Could you check a few things on this model? Use its own coordinates, in mm. A direction names the side the tool comes from. Give positions to 0.01 mm unless a question says otherwise; leave off trailing zeros. Order: outer loops, then holes, each group sorted by start corner. A loop starts at its lowest first (then second) coordinate and runs counter-clockwise, first axis right, second up. Notation, with made-up numbers: (23.25, -3.75) - (75.25, -3.75) arc R18 ccw to (75.25, 11.25) - close; hole circle Ø10 at (69, -0.75). An arc over 180 degrees is marked (long way). One line per question, with ' | ' between items. Start each with the question number.
1. If we mould it in two halves opening along X, with no side actions, what happens to faces 1 (the flat face through (5, -40, 5)), 2 (the flat face through (0, -12.5, 5)), 3 (the flat face through (0, -19, 10))? For each: released by +X, released by -X, zero draft, split by the parting line, or undercut.
2. Imagine slicing it at D-D (y = -54). Please give me the cut outline in (x, z), and give its area (3 significant figures).
3. Imagine slicing it at B-B (x = 0). Please give me the cut outline in (y, z), and give its area (3 significant figures).
4. Which directions (+Z, -Z, +X, -X, +Y, -Y) give clear straight access to the entire face, cutting with the end or side of a thin tool? Please do faces 4 (the flat face through (-5, -39, 5)), 5 (the flat face through (0, -59.365, 5)), 6 (the flat face through (2.5, -11, 5)).
5. I need wall thicknesses on probe 1 along Y at (x, z) = (0, 6.25); probe 2 along X at (y, z) = (-37.5, 9); probe 3 along X at (y, z) = (0, 6.25). Which ranges of each line are inside material? Lowest first, please. Write a range as from..to.
6. Imagine slicing it at C-C (z = 3.25). Please give me the cut outline in (x, y).
7. Imagine slicing it at A-A (y = 0). Please give me the cut outline in (x, z), and give its area (3 significant figures).
8. For P1, Ø6, axis at x = -14, z = 7.5, coming from the +Y side; P2, Ø0.8, axis at y = -11, z = 4, coming from the +X side; P3, Ø12, axis at x = 0, y = 0, coming from the +Z side; P4, Ø3, axis at y = -11, z = 4, coming from the -X side, each with a flat end and sliding along its axis, tell me the tip position at first contact or that it passes through.
```python
from build123d import *

# Parameters (mm, degrees)
BOSS_EXTRUDE1_DEPTH = 10


with BuildPart() as part:
    # Sketch1 → Boss-Extrude1 (new body)
    with BuildSketch(Plane.XY):
        with BuildLine():
            Line((-5, -59.364916731), (5, -59.364916731))
            Line((5, -59.364916731), (5, -19.364916731))
            ThreePointArc((5, -19.364916731), (0, 20), (-5, -19.364916731))
            Line((-5, -19.364916731), (-5, -59.364916731))
        make_face()
        with BuildLine():
            Line((-2.5, -12.5), (2.5, -12.5))
            Line((2.5, -12.5), (2.5, -9.682458366))
            ThreePointArc((2.5, -9.682458366), (0, 10), (-2.5, -9.682458366))
            Line((-2.5, -9.682458366), (-2.5, -12.5))
        make_face(mode=Mode.SUBTRACT)
    extrude(amount=BOSS_EXTRUDE1_DEPTH)


solid = part.part
```
Results found:
1) face 1: released by +X | face 2: undercut | face 3: zero draft
2) outline: (-5, 0) - (5, 0) - (5, 10) - (-5, 10) - close | area: 100 mm2
3) outline: (-59.36, 0) - (-12.5, 0) - (-12.5, 10) - (-59.36, 10) - close; (10, 0) - (20, 0) - (20, 10) - (10, 10) - close | area: 569 mm2
4) face 4: +Z, -Z, -X, -Y | face 5: +Z, -Z, +X, -X, -Y | face 6: +Z, -Z
5) probe 1: y = -59.36..-12.5, 10..20 | probe 2: x = -5..5 | probe 3: x = -20..-10, 10..20
6) outline: (-5, -59.36) - (5, -59.36) - (5, -19.36) arc R20 ccw (long way) to (-5, -19.36) - close; hole (-2.5, -12.5) - (2.5, -12.5) - (2.5, -9.68) arc R10 ccw (long way) to (-2.5, -9.68) - close
7) outline: (-20, 0) - (-10, 0) - (-10, 10) - (-20, 10) - close; (10, 0) - (20, 0) - (20, 10) - (10, 10) - close | area: 200 mm2
8) P1: stops at y = 16.7 | P2: stops at x = 16.96 | P3: passes through | P4: stops at x = -17.6
